```python
from build123d import *

# Parameters (mm, degrees)
CROQUIS1_W                   = 12.7
CROQUIS1_H                   = 5.8
SALIENTE_EXTRUIR1_DEPTH      = 3.3
CROQUIS2_W                   = 9.8
CROQUIS2_H                   = 0.9
SALIENTE_EXTRUIR2_DEPTH      = 8
REDONDEO1_R                  = 1
REDONDEO2_R                  = 1
CROQUIS3_W                   = 1.1
CROQUIS3_H                   = 5.8
CORTAR_EXTRUIR1_DEPTH        = 1
SALIENTE_EXTRUIR3_DEPTH      = 4
SALIENTE_EXTRUIR3_DEPTH_BACK = 9.9
CROQUIS4_W                   = 0.6
CROQUIS4_H                   = 0.6


with BuildPart() as part:
    # Croquis1 → Saliente-Extruir1 (new body)
    with BuildSketch(Plane(origin=(0, 0, 0), x_dir=(1, 0, 0), z_dir=(0, 1, 0))):
        Rectangle(CROQUIS1_W, CROQUIS1_H)
    extrude(amount=SALIENTE_EXTRUIR1_DEPTH)

    # Croquis2 → Saliente-Extruir2 (add)
    with BuildSketch(Plane(origin=(0, 3.3, 0), x_dir=(1, 0, 0), z_dir=(0, 1, 0))):
        with Locations((0, 2.45)):
            Rectangle(CROQUIS2_W, CROQUIS2_H)
    extrude(amount=SALIENTE_EXTRUIR2_DEPTH)

    # Redondeo1
    redondeo1_edges = [part.edges().sort_by_distance(p)[0] for p in [
        (4.9, 11.3, -2.45),
    ]]
    fillet(redondeo1_edges, radius=REDONDEO1_R)

    # Redondeo2
    redondeo2_edges = [part.edges().sort_by_distance(p)[0] for p in [
        (-4.9, 11.3, -2.45),
    ]]
    fillet(redondeo2_edges, radius=REDONDEO2_R)

    # Croquis3 → Cortar-Extruir1 (cut)
    with BuildSketch(Plane.XZ):
        with Locations((-5, 0)):
            Rectangle(CROQUIS3_W, CROQUIS3_H)
        with Locations((-2.5, 0)):
            Rectangle(CROQUIS3_W, CROQUIS3_H)
        Rectangle(CROQUIS3_W, CROQUIS3_H)
        with Locations((2.5, 0)):
            Rectangle(CROQUIS3_W, CROQUIS3_H)
        with Locations((5, 0)):
            Rectangle(CROQUIS3_W, CROQUIS3_H)
    extrude(amount=-CORTAR_EXTRUIR1_DEPTH, mode=Mode.SUBTRACT)

    # Croquis4 → Saliente-Extruir3 (add, two sides: drawn at the far end of the back side and taken through both)
    with BuildSketch(Plane(origin=(0, 1, 0), x_dir=(-1, 0, 0), z_dir=(0, -1, 0)).offset(-SALIENTE_EXTRUIR3_DEPTH_BACK)):
        with Locations((5, 0.5)):
            Rectangle(CROQUIS4_W, CROQUIS4_H)
        with Locations((2.5, 0.5)):
            Rectangle(CROQUIS4_W, CROQUIS4_H)
        with Locations((0, 0.5)):
            Rectangle(CROQUIS4_W, CROQUIS4_H)
        with Locations((-2.5, 0.5)):
            Rectangle(CROQUIS4_W, CROQUIS4_H)
        with Locations((-5, 0.5)):
            Rectangle(CROQUIS4_W, CROQUIS4_H)
    extrude(amount=SALIENTE_EXTRUIR3_DEPTH + SALIENTE_EXTRUIR3_DEPTH_BACK)


solid = part.part
```
Geometry: final body of the model. Coordinates: model frame, mm. A direction names the side the tool comes from. Round coordinates to 2 decimals unless told otherwise and drop trailing zeros. Order: outer loops, then holes, each group sorted by start corner. A loop starts at its lowest first (then second) coordinate and runs counter-clockwise, first axis right, second up. Notation, with made-up numbers: (-21.5, 1.5) -> (-15.5, 1.5) arc R7 ccw to (-15.5, 14.5) -> close; hole circle Ø8 at (-2.75, -23). An arc over 180 degrees is marked (long way). Use one line per item in the form item = value. Start each with the question number.
1. Cut plane D-D (y = 0.75). Count the separate pieces of the cut face and the enclosed holes in it, then the cut area to 3 significant figures.
2. Pin query (flat end, axial travel): pin 1 Ø1.5 at (x, z) = (1, -0.5) entering from -Y; pin 2 Ø0.5 at (x, z) = (-5, -0.5) entering from +Y; pin 3 Ø0.7 at (x, y) = (-5, 5.5) entering from +Z; pin 4 Ø0.9 at (x, z) = (5, 1) entering from -Y. Return the tip coordinate at first contact, or that it passes through.
3. Cut plane B-B (y = 5.5). Return the cut outline in (x, z), then the cut area to 3 significant figures.
4. Cut plane A-A (z = 1.35). Return the cut outline in (x, y).
5. Reachability of faces 1 (the face through (-4.599, 11.015, -2.456)), 2 (the face through (-0.1, 11.3, -2.5)), 3 (the face through (-4.45, 0.5, 0)) from +Z, -Z, +X, -X, +Y, -Y: full face, straight path, thin tool, end or side. Return the list, or none.
6. Line query: probe 1 along X at (y, z) = (4, -0.45); probe 2 along Z at (x, y) = (-2.75, 9); probe 3 along Z at (x, y) = (4.5, 4.5). Output: solid intervals per line, ascending.
7. Draft query along X for faces 4 (the face through (0, 7, -2)), 5 (the face through (0, 1, 0)), 6 (the face through (6.35, 2, 0)). Return one class per face: pulls with the +X half, pulls with the -X half, needs draft (parallel to the pull), parting line crosses it, or undercut.
8. Cut plane C-C (x = 1). Return the cut outline in (y, z).
Solution:
q1.separate_pieces = 11
q1.enclosed_holes = 0
q1.area = 43.6 mm^2
q2.pin_1 = -3
q2.pin_2 = 10.9
q2.pin_3 = -0.2
q2.pin_4 = 1
q3.outline = (-5.3, -0.8) -> (-4.7, -0.8) -> (-4.7, -0.2) -> (-5.3, -0.2) -> close; (-4.9, -2.9) -> (4.9, -2.9) -> (4.9, -2) -> (-4.9, -2) -> close; (-2.8, -0.8) -> (-2.2, -0.8) -> (-2.2, -0.2) -> (-2.8, -0.2) -> close; (-0.3, -0.8) -> (0.3, -0.8) -> (0.3, -0.2) -> (-0.3, -0.2) -> close; (2.2, -0.8) -> (2.8, -0.8) -> (2.8, -0.2) -> (2.2, -0.2) -> close; (4.7, -0.8) -> (5.3, -0.8) -> (5.3, -0.2) -> (4.7, -0.2) -> close
q3.area = 10.6 mm^2
q4.outline = (-6.35, 0) -> (-5.55, 0) -> (-5.55, 1) -> (-4.45, 1) -> (-4.45, 0) -> (-3.05, 0) -> (-3.05, 1) -> (-1.95, 1) -> (-1.95, 0) -> (-0.55, 0) -> (-0.55, 1) -> (0.55, 1) -> (0.55, 0) -> (1.95, 0) -> (1.95, 1) -> (3.05, 1) -> (3.05, 0) -> (4.45, 0) -> (4.45, 1) -> (5.55, 1) -> (5.55, 0) -> (6.35, 0) -> (6.35, 3.3) -> (-6.35, 3.3) -> close
q5.face_1 = -Z, -X, +Y
q5.face_2 = +Z, -Z, +X, -X, +Y
q5.face_3 = +Z, -Z, -Y
q6.probe_1 = -5.3 to -4.7, -2.8 to -2.2, -0.3 to 0.3, 2.2 to 2.8, 4.7 to 5.3
q6.probe_2 = -2.9 to -2, -0.8 to -0.2
q6.probe_3 = -2.9 to -2
q7.face_4 = needs draft
q7.face_5 = undercut
q7.face_6 = pulls with the +X half
q8.outline = (0, -2.9) -> (11.3, -2.9) -> (11.3, -2) -> (3.3, -2) -> (3.3, 2.9) -> (0, 2.9) -> close
